Geometry: final body of the model. Coordinates: model frame, mm. A direction names the side the tool comes from. Give positions to 0.01 mm unless a question says otherwise; leave off trailing zeros. Order: outer loops, then holes, each group sorted by start corner. A loop starts at its lowest first (then second) coordinate and runs counter-clockwise, first axis right, second up. Notation, with made-up numbers: M 74,24 L 98,24 A27 ccw 98,59 Z; hole C 10,-28.75 d1. An arc over 180 degrees is marked long. Use CSV: the item, a comma, the result in double quotes.
```python
from build123d import *

# Parameters (mm, degrees)
F1_DEPTH = 1
F3_DEPTH = 12.5
F4_R     = 0.3
F5_DEPTH = 8
F6_SIZE2 = 5
F6_SIZE  = 0.2
F7_R     = 0.1


with BuildPart() as f1:
    # F0 (on Right) → F1 (new body, symmetric)
    with BuildSketch(Plane.YZ):
        Polygon((1.6081985701, 24.68570705), (-6.6278126925, 24.68570705), (-6.6278126925, 23.64570705), (0, 23.64570705), (-2.7713922732, 0.7310225915), (-5.147449191, 6.8627829807), (-8.647449191, 6.8627829807), (-2.4741467328, -9.0683216995), align=None)
    extrude(amount=F1_DEPTH, both=True)

    # F2 (on face) → F3 (cut, symmetric)
    with BuildSketch(Plane(origin=(0, -1.3575309583, 0.1641851458), x_dir=(-1, 0, 0), z_dir=(0, 0.9927655515, -0.1200689795))):
        Polygon((-0.5489893374, -11.4567056298), (-1, 24.7002143338), (-8.0727264285, 24.7002143338), (-7.1800793521, -14.4110620022), (7.0385080762, -14.4110620022), (7.0385080762, 24.0597836673), (1, 24.7002143338), (0.4711783549, -11.4567056298), align=None)
    extrude(amount=F3_DEPTH, both=True, mode=Mode.SUBTRACT)

    # F4 (on face) → F5 (join)
    with BuildSketch(Plane.XZ.offset(6.6278126925)):
        with Locations((0.0010640627, 24.16570705)):
            Circle(F4_R)
    extrude(amount=F5_DEPTH)

    # F6
    f6_edges = [f1.edges().sort_by_distance(p)[0] for p in [
        (-0.298936, -14.627813, 24.165707),
    ]]
    f6_side = f1.faces().sort_by_distance((0.001064, -14.627813, 24.165707))[0]
    chamfer(f6_edges, length=F6_SIZE, length2=F6_SIZE2, reference=f6_side)

    # F7
    f7_edges = [f1.edges().sort_by_distance(p)[0] for p in [
        (0.732986, -3.959421, 3.796903),
        (-0.992768, -2.509807, 24.685707),
        (-0.813282, -1.385696, 12.188365),
        (0.766552, -6.897449, 6.862783),
        (0.993832, -2.509807, 24.685707),
        (-0.612964, -5.560798, -1.102769),
        (0.840756, -1.385696, 12.188365),
        (0.979749, -3.313906, 23.645707),
        (0.669912, -5.560798, -1.102769),
        (0.787947, -0.432974, 7.808693),
        (-0.726276, -6.897449, 6.862783),
        (0, 1.608199, 24.685707),
        (-0.298936, -9.627813, 24.165707),
        (-0.751362, -0.432974, 7.808693),
        (-0.686919, -3.959421, 3.796903),
        (0.002175, -6.627813, 23.645707),
        (0.981225, -6.627813, 24.165707),
        (0.001319, 0, 23.645707),
        (0.026155, -2.771392, 0.731023),
        (-0.977986, -6.627813, 24.165707),
        (0.020364, -8.647449, 6.862783),
        (0.036585, -2.474147, -9.068322),
        (0.019912, -5.147449, 6.862783),
        (0.001064, -6.627813, 24.685707),
        (-0.976256, -3.313906, 23.645707),
    ]]
    fillet(f7_edges, radius=F7_R)


solid = f1.part
```
1. Pull-direction query (Y, two-part tool) for faces 1 (the face through (0, -7, 6.863)), 2 (the face through (0, 0, 11.4)), 3 (the face through (0, -4, 3.9)); classes: +Y half, -Y half, draft (parallel to the pull), parting line (faces both ways), or undercut.
Answer:
face 1,"draft"
face 2,"+Y half"
face 3,"undercut"
2. Section A-A, the plane y = -9.25. Return the cut outline in (x, z), plus the area to 3 significant figures.
Answer:
outline,"C 0,24.17 d0.6"
area,"0.283 mm2"
3. Line query: line 1 (X direction, y = -5.5, z = -1); line 2 (Y direction, x = -0.35, z = 2.5); line 3 (Z direction, x = 0, y = -13.75). Output: solid intervals per line, ascending.
Answer:
line 1,"-0.61 to 0.67"
line 2,"-6.96 to -3.46, -2.56 to -1.08"
line 3,"24.03 to 24.3"
4. Reachability of faces 4 (the face through (0.029, -5.649, -0.876)), 5 (the face through (0.01, -1.35, 12.49)), 6 (the face through (0, -3, 23.646)) from +Z, -Z, +X, -X, +Y, -Y: full face, straight path, thin tool, end or side. Return the list, or none.
Answer:
face 4,"-Z, +X, -X, -Y"
face 5,"+X, -X"
face 6,"+X, -X, -Y"
5. Pin query (flat end, axial travel): pin 1 Ø5 at (y, z) = (-3, 7.5) entering from +X; pin 2 Ø2 at (y, z) = (-1.5, 7.5) entering from -X. Return the tip coordinate at first contact, or that it passes through.
Answer:
pin 1,"x = 0.81"
pin 2,"x = -0.76"
